The listing builds one solid part. Answer for the finished solid, in the listing's coordinates (mm). A direction names the side the tool comes from. Round coordinates to 2 decimals unless told otherwise and drop trailing zeros. Write each loop counter-clockwise with the first axis right and the second up, starting at its lowest first coordinate (ties: lowest second). Pieces come first, ordered by that corner, then holes. Notation, with made-up numbers: (28.5, 65.5) - (51.5, 65.5) arc R14 ccw to (51.5, 86.5) - close; hole circle Ø10 at (-28.75, -29). An arc over 180 degrees is marked (long way). Return JSON: item names as keys, results as strings. Group by question number.
from build123d import *

# Parameters (mm, degrees)
BASE_FLANGE1_DEPTH       = 1
SKETCHED_START           = 11.616422755
SKETCHED_BEND1_OUTLINE_W = 40
SKETCHED_BEND1_OUTLINE_H = 1
SKETCHED_BEND1_DEPTH     = 28.383577245
SKETCHED_START_2         = 10.821902755
SKETCHED_BEND1_2_DEPTH   = 0.00548
SKETCHED_START_3         = 9.821902755
SKETCHED_BEND1_3_DEPTH   = 2
SKETCHED_START_4         = -20
SKETCHED_BEND1_4_DEPTH   = 40
SKETCH7_R                = 2.025
CUT_EXTRUDE1_DEPTH       = 10
F_6_CLEARANCE_HOLE1_D    = 3.7973
F_4_CLEARANCE_HOLE2_D    = 3.2639


with BuildPart() as part:
    # Base-Flange1: sheet metal written as solids
    # Sketch1 → Base-Flange1 (new body)
    with BuildSketch(Plane(origin=(0, 0, 0), x_dir=(1, 0, 0), z_dir=(0, 1, 0))):
        with BuildLine():
            Line((-20, -8), (-20, -35))
            ThreePointArc((-20, -35), (-18.535533906, -38.535533906), (-15, -40))
            Line((-15, -40), (15, -40))
            ThreePointArc((15, -40), (18.535533906, -38.535533906), (20, -35))
            Line((20, -35), (20, -8))
            Line((20, -8), (26, -8))
            ThreePointArc((26, -8), (27.414213562, -7.414213562), (28, -6))
            Line((28, -6), (28, 6))
            ThreePointArc((28, 6), (27.414213562, 7.414213562), (26, 8))
            Line((26, 8), (20, 8))
            Line((20, 8), (20, 25))
            ThreePointArc((20, 25), (15.606601718, 35.606601718), (5, 40))
            Line((5, 40), (-5, 40))
            ThreePointArc((-5, 40), (-15.606601718, 35.606601718), (-20, 25))
            Line((-20, 25), (-20, 8))
            Line((-20, 8), (-26, 8))
            ThreePointArc((-26, 8), (-27.414213562, 7.414213562), (-28, 6))
            Line((-28, 6), (-28, -6))
            ThreePointArc((-28, -6), (-27.414213562, -7.414213562), (-26, -8))
            Line((-26, -8), (-20, -8))
        make_face()
    extrude(amount=-BASE_FLANGE1_DEPTH)

    # Sketched Bend1: read off the stored shape, not the designer's step
    # Sketched Bend1 outline → Sketched Bend1 (cut)
    with BuildSketch(Plane.XY.offset(SKETCHED_START)):
        with Locations((0, -0.5)):
            Rectangle(SKETCHED_BEND1_OUTLINE_W, SKETCHED_BEND1_OUTLINE_H)
    extrude(amount=SKETCHED_BEND1_DEPTH, mode=Mode.SUBTRACT)

    # Sketched Bend1 2 outline → Sketched Bend1 2 (add)
    with BuildSketch(Plane.XY.offset(SKETCHED_START_2)):
        with BuildLine():
            Line((20, 0), (20, 23.821902755))
            ThreePointArc((20, 23.821902755), (18.535533906, 27.357436661), (15, 28.821902755))
            Line((15, 28.821902755), (-15, 28.821902755))
            ThreePointArc((-15, 28.821902755), (-18.535533906, 27.357436661), (-20, 23.821902755))
            Line((-20, 23.821902755), (-20, 0))
            Line((-20, 0), (20, 0))
        make_face()
    extrude(amount=SKETCHED_BEND1_2_DEPTH)

    # Sketched Bend1 3 outline → Sketched Bend1 3 (add)
    with BuildSketch(Plane.XY.offset(SKETCHED_START_3)):
        with BuildLine():
            Line((20, 0), (20, 23.821902755))
            ThreePointArc((20, 23.821902755), (18.535533906, 27.357436661), (15, 28.821902755))
            Line((15, 28.821902755), (-15, 28.821902755))
            ThreePointArc((-15, 28.821902755), (-18.535533906, 27.357436661), (-20, 23.821902755))
            Line((-20, 23.821902755), (-20, 0))
            Line((-20, 0), (20, 0))
        make_face()
    extrude(amount=SKETCHED_BEND1_3_DEPTH)

    # Sketched Bend1 4 outline → Sketched Bend1 4 (cut)
    with BuildSketch(Plane.YZ.offset(SKETCHED_START_4)):
        with BuildLine():
            Line((28.821902755, 9.821902755), (28.821902755, 10.821902755))
            Line((28.821902755, 10.821902755), (1, 10.821902755))
            ThreePointArc((1, 10.821902755), (0.292893219, 10.529009536), (0, 9.821902755))
            Line((0, 9.821902755), (28.821902755, 9.821902755))
        make_face()
        with BuildLine():
            ThreePointArc((-1, 9.821902755), (-0.414213562, 11.236116317), (1, 11.821902755))
            Line((1, 11.821902755), (0, 11.821902755))
            Line((0, 11.821902755), (0, 11.616422755))
            Line((0, 11.616422755), (-1, 11.616422755))
            Line((-1, 11.616422755), (-1, 9.821902755))
        make_face()
    extrude(amount=SKETCHED_BEND1_4_DEPTH, mode=Mode.SUBTRACT)

    # Sketch7 → Cut-Extrude1 (cut)
    with BuildSketch(Plane(origin=(0, 0, 0), x_dir=(1, 0, 0), z_dir=(0, 1, 0))):
        with Locations(Location((0, 32.178097245, 0), (0, 0, 270))):
            Circle(SKETCH7_R)
    extrude(amount=-CUT_EXTRUDE1_DEPTH, mode=Mode.SUBTRACT)

    # #6 Clearance Hole1 (through all)
    with Locations(Plane(origin=(0, 0, 10.821902755), x_dir=(-1, 0, 0), z_dir=(0, 0, -1))):
        with Locations((13, 13.821902755), (-13, 13.821902755), (0, 23.821902755)):
            Hole(F_6_CLEARANCE_HOLE1_D / 2)

    # #4 Clearance Hole2 (through all)
    with Locations(Plane(origin=(0, 0, 0), x_dir=(1, 0, 0), z_dir=(0, 1, 0))):
        with Locations((-24, 4), (-24, -4), (24, 4), (24, -4)):
            Hole(F_4_CLEARANCE_HOLE2_D / 2)


solid = part.part
(1) Find section B-B (x = -13). Write down the section's boundary in (y, z).
(2) For faces 1 (the cylindrical face through (27.4, -0.49, 7.43)), 2 (the flat face through (0, 0, -10)), determine the directions among +Z, -Z, +X, -X, +Y, -Y from which every point of the face is accessible in a straight line to the end or side of a thin tool.
(3) Determine the mould class of faces 3 (the cylindrical face through (-18.496, 27.396, 11.315)), 4 (the flat face through (0, 15, 10.822)), 5 (the cylindrical face through (11.49, 12.67, 11.33)), 6 (the cylindrical face through (27.43, -0.49, -7.4)) for opening direction X: +X half, -X half, draft (parallel to the pull), parting line (faces both ways), or undercut.
(4) Find section C-C (y = 15). Write down the section's boundary in (x, z), plus the area to 3 significant figures.
(5) Flat-ended cylindrical pins translate along their axes: pin 1 (3 mm diameter, centred on y = 17.5, z = 11, fed in from +X); pin 2 (0.5 mm diameter, centred on x = 24.5, y = -0.5, fed in from +Z); pin 3 (0.8 mm diameter, centred on x = 24.5, y = -0.5, fed in from -Z); pin 4 (3 mm diameter, centred on x = 21, y = 11, fed in from +Z). Find the tip coordinate at first contact, or state that the pin passes through.
(6) Find section A-A (z = -4). Write down the section's boundary in (x, y), plus the area to 3 significant figures.
(7) Find section D-D (z = -31). Write down the section's boundary in (x, y).
(8) Consider line 1 (Z direction, x = -24, y = -0.75); line 2 (X direction, y = -0.35, z = 4); line 3 (Y direction, x = 12, z = -2.5). Determine where each line is inside the solid, lowest interval first.
Check sheet entries:
{
 "1": {"outline": "(-1, -37.69) - (0, -37.69) - (0, 9.82) arc R1 cw to (1, 10.82) - (11.92, 10.82) - (11.92, 11.82) - (1, 11.82) arc R2 ccw to (-1, 9.82) - close; (15.72, 10.82) - (28.82, 10.82) - (28.82, 11.82) - (15.72, 11.82) - close"},
 "2": {"face 1": "+Z, +X, +Y, -Y", "face 2": "-Z, +X, -X, +Y"},
 "3": {"face 3": "-X half", "face 4": "draft", "face 5": "undercut", "face 6": "+X half"},
 "4": {"outline": "(-20, 10.82) - (-14.49, 10.82) - (-14.49, 11.82) - (-20, 11.82) - close; (-11.51, 10.82) - (11.51, 10.82) - (11.51, 11.82) - (-11.51, 11.82) - close; (14.49, 10.82) - (20, 10.82) - (20, 11.82) - (14.49, 11.82) - close", "area": "34.0 mm^2"},
 "5": {"pin 1": "stops at x = 20", "pin 2": "stops at z = 8", "pin 3": "stops at z = -8", "pin 4": "stops at z = 11.82"},
 "6": {"outline": "(-28, -1) - (-25.63, -1) - (-25.63, 0) - (-28, 0) - close; (-22.37, -1) - (22.37, -1) - (22.37, 0) - (-22.37, 0) - close; (25.63, -1) - (28, -1) - (28, 0) - (25.63, 0) - close", "area": "49.5 mm^2"},
 "7": {"outline": "(-18.75, -1) - (-1.65, -1) - (-1.65, 0) - (-18.75, 0) - close; (1.65, -1) - (18.75, -1) - (18.75, 0) - (1.65, 0) - close"},
 "8": {"line 1": "z = -8 to -5.63, -2.37 to 2.37, 5.63 to 8", "line 2": "x = -28 to -25.63, -22.37 to 22.37, 25.63 to 28", "line 3": "y = -1 to 0"}
}
